from build123d import *

# Parameters (mm, degrees)
SKETCH8_W                       = 35
SKETCH8_H                       = 30
BOSS_EXTRUDE7_DEPTH             = 80
SKETCH10_R                      = 16.5
CUT_EXTRUDE3_DEPTH              = 18.5
CUT_EXTRUDE3_DEPTH_BACK         = 18.5
SKETCH11_W                      = 38.336381606
SKETCH11_H                      = 16.50007926
CUT_EXTRUDE4_DEPTH              = 18.5
CUT_EXTRUDE4_DEPTH_BACK         = 18.5
SKETCH12_W                      = 33.824881692
SKETCH12_H                      = 15
CUT_EXTRUDE5_DEPTH              = 18.5
CUT_EXTRUDE5_DEPTH_BACK         = 18.5
SKETCH13_W                      = 45.541829225
SKETCH13_H                      = 41.48776408
CUT_EXTRUDE6_DEPTH              = 18.5
CUT_EXTRUDE6_DEPTH_BACK         = 18.5
SKETCH15_W                      = 35
SKETCH15_H                      = 7.5
BOSS_EXTRUDE9_DEPTH             = 2
CUT_EXTRUDE7_DEPTH              = 2
SKETCH18_R                      = 3.2
CUT_EXTRUDE10_DEPTH             = 9.24996037
CUT_EXTRUDE10_DEPTH_BACK        = 6.4
CUT_EXTRUDE11_REACH             = 10.25
SKETCH19_R                      = 3.4
CUT_EXTRUDE11_DIRECTION_2_DEPTH = 4.9


with BuildPart() as part:
    # Sketch8 → Boss-Extrude7 (new body)
    with BuildSketch(Plane(origin=(0, 0, 0), x_dir=(1, 0, 0), z_dir=(0, 1, 0))):
        Rectangle(SKETCH8_W, SKETCH8_H)
    extrude(amount=BOSS_EXTRUDE7_DEPTH)

    # Sketch10 → Cut-Extrude3 (cut, two sides)
    with BuildSketch(Plane(origin=(0, 0, 0), x_dir=(0, 0, -1), z_dir=(1, 0, 0))) as cut_extrude3_sk:
        with Locations((0, 40)):
            Circle(SKETCH10_R)
    extrude(amount=CUT_EXTRUDE3_DEPTH, mode=Mode.SUBTRACT)
    extrude(cut_extrude3_sk.sketch, amount=-CUT_EXTRUDE3_DEPTH_BACK, mode=Mode.SUBTRACT)

    # Sketch11 → Cut-Extrude4 (cut, two sides)
    with BuildSketch(Plane(origin=(0, 0, 0), x_dir=(0, 0, -1), z_dir=(1, 0, 0))) as cut_extrude4_sk:
        with Locations((0, 40)):
            Rectangle(SKETCH11_W, SKETCH11_H)
    extrude(amount=CUT_EXTRUDE4_DEPTH, mode=Mode.SUBTRACT)
    extrude(cut_extrude4_sk.sketch, amount=-CUT_EXTRUDE4_DEPTH_BACK, mode=Mode.SUBTRACT)

    # Sketch12 → Cut-Extrude5 (cut, two sides)
    with BuildSketch(Plane(origin=(0, 0, 0), x_dir=(0, 0, -1), z_dir=(1, 0, 0))) as cut_extrude5_sk:
        with Locations((0.439040256, 7.5)):
            Rectangle(SKETCH12_W, SKETCH12_H)
    extrude(amount=CUT_EXTRUDE5_DEPTH, mode=Mode.SUBTRACT)
    extrude(cut_extrude5_sk.sketch, amount=-CUT_EXTRUDE5_DEPTH_BACK, mode=Mode.SUBTRACT)

    # Sketch13 → Cut-Extrude6 (cut, two sides)
    with BuildSketch(Plane(origin=(0, 0, 0), x_dir=(0, 0, -1), z_dir=(1, 0, 0))) as cut_extrude6_sk:
        with Locations((-6.569234617, 60.808180877)):
            Rectangle(SKETCH13_W, SKETCH13_H)
    extrude(amount=CUT_EXTRUDE6_DEPTH, mode=Mode.SUBTRACT)
    extrude(cut_extrude6_sk.sketch, amount=-CUT_EXTRUDE6_DEPTH_BACK, mode=Mode.SUBTRACT)

    # Sketch15 → Boss-Extrude9 (add)
    with BuildSketch(Plane(origin=(0, 15, 0), x_dir=(-1, 0, 0), z_dir=(0, -1, 0))):
        with Locations((0, -18.75)):
            Rectangle(SKETCH15_W, SKETCH15_H)
        with Locations((0, 18.75)):
            Rectangle(SKETCH15_W, SKETCH15_H)
    extrude(amount=-BOSS_EXTRUDE9_DEPTH)

    # Sketch16 → Cut-Extrude7 (cut)
    with BuildSketch(Plane(origin=(0, 15, 0), x_dir=(-1, 0, 0), z_dir=(0, -1, 0))):
        with BuildLine():
            Line((10, -20.863517543), (-10, -20.863517543))
            ThreePointArc((-10, -20.863517543), (-12, -18.863517543), (-10, -16.863517543))
            Line((-10, -16.863517543), (10, -16.863517543))
            ThreePointArc((10, -16.863517543), (12, -18.863517543), (10, -20.863517543))
        make_face()
        with BuildLine():
            Line((10, 16.803450623), (-10, 16.803450623))
            ThreePointArc((-10, 16.803450623), (-12, 18.803450623), (-10, 20.803450623))
            Line((-10, 20.803450623), (10, 20.803450623))
            ThreePointArc((10, 20.803450623), (12, 18.803450623), (10, 16.803450623))
        make_face()
    extrude(amount=-CUT_EXTRUDE7_DEPTH, mode=Mode.SUBTRACT)

    # Sketch18 → Cut-Extrude10 (cut, two sides)
    with BuildSketch(Plane(origin=(0, 23.5, 0), x_dir=(1, 0, 0), z_dir=(0, 1, 0))) as cut_extrude10_sk:
        Circle(SKETCH18_R)
        with Locations((10, 0)):
            Circle(SKETCH18_R)
        with Locations((-10, 0)):
            Circle(SKETCH18_R)
    extrude(amount=CUT_EXTRUDE10_DEPTH, mode=Mode.SUBTRACT)
    extrude(cut_extrude10_sk.sketch, amount=-CUT_EXTRUDE10_DEPTH_BACK, mode=Mode.SUBTRACT)

    # Sketch19 → Cut-Extrude11 (cut, up to next)
    with BuildSketch(Plane(origin=(0, 23.5, 0), x_dir=(1, 0, 0), z_dir=(0, 1, 0)), mode=Mode.PRIVATE) as cut_extrude11_sk1:
        with Locations((-10, -10)):
            Circle(SKETCH19_R)
    cut_extrude11_tool1 = extrude(cut_extrude11_sk1.sketch, amount=CUT_EXTRUDE11_REACH, mode=Mode.PRIVATE) & part.part
    add(cut_extrude11_tool1.solids().sort_by_distance((-10, 23.5, 10))[0], mode=Mode.SUBTRACT)
    # Sketch19 → Cut-Extrude11 (cut, up to next)
    with BuildSketch(Plane(origin=(0, 23.5, 0), x_dir=(1, 0, 0), z_dir=(0, 1, 0)), mode=Mode.PRIVATE) as cut_extrude11_sk2:
        with Locations((0, -10)):
            Circle(SKETCH19_R)
    cut_extrude11_tool2 = extrude(cut_extrude11_sk2.sketch, amount=CUT_EXTRUDE11_REACH, mode=Mode.PRIVATE) & part.part
    add(cut_extrude11_tool2.solids().sort_by_distance((0, 23.5, 10))[0], mode=Mode.SUBTRACT)
    # Sketch19 → Cut-Extrude11 (cut, up to next)
    with BuildSketch(Plane(origin=(0, 23.5, 0), x_dir=(1, 0, 0), z_dir=(0, 1, 0)), mode=Mode.PRIVATE) as cut_extrude11_sk3:
        with Locations((10, -10)):
            Circle(SKETCH19_R)
    cut_extrude11_tool3 = extrude(cut_extrude11_sk3.sketch, amount=CUT_EXTRUDE11_REACH, mode=Mode.PRIVATE) & part.part
    add(cut_extrude11_tool3.solids().sort_by_distance((10, 23.5, 10))[0], mode=Mode.SUBTRACT)
    # Sketch19 → Cut-Extrude11 (cut, up to next)
    with BuildSketch(Plane(origin=(0, 23.5, 0), x_dir=(1, 0, 0), z_dir=(0, 1, 0)), mode=Mode.PRIVATE) as cut_extrude11_sk4:
        with Locations((-10, 10)):
            Circle(SKETCH19_R)
    cut_extrude11_tool4 = extrude(cut_extrude11_sk4.sketch, amount=CUT_EXTRUDE11_REACH, mode=Mode.PRIVATE) & part.part
    add(cut_extrude11_tool4.solids().sort_by_distance((-10, 23.5, -10))[0], mode=Mode.SUBTRACT)
    # Sketch19 → Cut-Extrude11 (cut, up to next)
    with BuildSketch(Plane(origin=(0, 23.5, 0), x_dir=(1, 0, 0), z_dir=(0, 1, 0)), mode=Mode.PRIVATE) as cut_extrude11_sk5:
        with Locations((0, 10)):
            Circle(SKETCH19_R)
    cut_extrude11_tool5 = extrude(cut_extrude11_sk5.sketch, amount=CUT_EXTRUDE11_REACH, mode=Mode.PRIVATE) & part.part
    add(cut_extrude11_tool5.solids().sort_by_distance((0, 23.5, -10))[0], mode=Mode.SUBTRACT)
    # Sketch19 → Cut-Extrude11 (cut, up to next)
    with BuildSketch(Plane(origin=(0, 23.5, 0), x_dir=(1, 0, 0), z_dir=(0, 1, 0)), mode=Mode.PRIVATE) as cut_extrude11_sk6:
        with Locations((10, 10)):
            Circle(SKETCH19_R)
    cut_extrude11_tool6 = extrude(cut_extrude11_sk6.sketch, amount=CUT_EXTRUDE11_REACH, mode=Mode.PRIVATE) & part.part
    add(cut_extrude11_tool6.solids().sort_by_distance((10, 23.5, -10))[0], mode=Mode.SUBTRACT)

    # Sketch19 → Cut-Extrude11 direction 2 (cut)
    with BuildSketch(Plane(origin=(0, 23.5, 0), x_dir=(1, 0, 0), z_dir=(0, 1, 0))):
        with Locations((-10, -10)):
            Circle(SKETCH19_R)
        with Locations((0, -10)):
            Circle(SKETCH19_R)
        with Locations((10, -10)):
            Circle(SKETCH19_R)
        with Locations((-10, 10)):
            Circle(SKETCH19_R)
        with Locations((0, 10)):
            Circle(SKETCH19_R)
        with Locations((10, 10)):
            Circle(SKETCH19_R)
    extrude(amount=-CUT_EXTRUDE11_DIRECTION_2_DEPTH, mode=Mode.SUBTRACT)


solid = part.part
The listing builds one solid part. Answer for the finished solid, in the listing's coordinates (mm). A direction names the side the tool comes from. Give positions to 0.01 mm unless a question says otherwise; leave off trailing zeros. Loops run counter-clockwise (first coordinate to the right, second up) from the corner with the lowest first, then second, coordinate; pieces in that order, holes last.
Item 1: Each of these flat-tipped pins is pushed along its axis until it touches: pin 1 Ø1.9 at (x, z) = (-11, -1.5) entering from +Y; pin 2 Ø1 at (x, z) = (6, 1) entering from +Y; pin 3 Ø6 at (x, z) = (-6.5, 20) entering from +Y. Where does it stop, or does it pass through?
Derived:
pin 1: stops at y = 17.1
pin 2: stops at y = 23.57
pin 3: stops at y = 17
Item 2: A cutting plane is placed at A-A (x = -5.5). Give the vertices of the cut face in (y, z).
Derived:
outline: (15, -22.5) - (17, -22.5) - (17, -20.8) - (15, -20.8) - close; (15, -16.8) - (17, -16.8) - (17, -15) - (31.75, -15) - (31.75, -14.29) arc R16.5 cw to (31.75, 14.29) - (31.75, 15) - (17, 15) - (17, 16.86) - (15, 16.86) - close; (15, 20.86) - (17, 20.86) - (17, 22.5) - (15, 22.5) - close
Item 3: Determine the mould class of faces 1 (the flat face through (-17.5, 21, -5)), 2 (the flat face through (0, 16, 20.864)), 3 (the flat face through (0, 16, 22.5)) for opening direction X: +X half, -X half, draft (parallel to the pull), parting line (faces both ways), or undercut.
Derived:
face 1: -X half
face 2: undercut
face 3: draft
Item 4: A tool of negligible diameter and unlimited length cuts with its end or side. For faces 4 (the cylindrical face through (-12, 16, 18.8)), 5 (the flat face through (0, 17, 16)), 6 (the flat face through (-10, 18.6, 10)), from which of +Z, -Z, +X, -X, +Y, -Y can it reach the whole face along a straight path? Write none if from no direction.
Derived:
face 4: +Y, -Y
face 5: +Z, +X, -X, +Y
face 6: +Y
Item 5: A cutting plane is placed at D-D (z = -1.5). Give the vertices of the cut face in (x, y).
Derived:
outline: (-17.5, 15) - (17.5, 15) - (17.5, 23.57) - (12.83, 23.57) - (12.83, 17.1) - (7.17, 17.1) - (7.17, 23.57) - (2.83, 23.57) - (2.83, 17.1) - (-2.83, 17.1) - (-2.83, 23.57) - (-7.17, 23.57) - (-7.17, 17.1) - (-12.83, 17.1) - (-12.83, 23.57) - (-17.5, 23.57) - close
Item 6: A cutting plane is placed at B-B (y = 24.75). Give the vertices of the cut face in (x, z).
Derived:
outline: (-17.5, -15) - (17.5, -15) - (17.5, -6.3) - (-17.5, -6.3) - close; (-17.5, 6.3) - (17.5, 6.3) - (17.5, 15) - (-17.5, 15) - close; hole circle Ø6.8 at (-10, -10); hole circle Ø6.8 at (-10, 10); hole circle Ø6.8 at (0, -10); hole circle Ø6.8 at (0, 10); hole circle Ø6.8 at (10, -10); hole circle Ø6.8 at (10, 10)
Item 7: Find the intervals of material crossed by line 1 along Z through (x, y) = (0, 22.3); line 2 along X through (y, z) = (25, -10); line 3 along X through (y, z) = (19.75, 0), in increasing order.
Derived:
line 1: z = -15 to -13.4, -6.6 to -3.2, 3.2 to 6.6, 13.4 to 15
line 2: x = -17.5 to -13.4, -6.6 to -3.4, 3.4 to 6.6, 13.4 to 17.5
line 3: x = -17.5 to -13.2, -6.8 to -3.2, 3.2 to 6.8, 13.2 to 17.5
Item 8: A cutting plane is placed at C-C (y = 29.25). Give the vertices of the cut face in (x, z), then the cut area to 3 significant figures.
Derived:
outline: (-17.5, -15) - (17.5, -15) - (17.5, -12.52) - (12.29, -12.52) arc R3.4 cw to (7.71, -12.52) - (2.29, -12.52) arc R3.4 cw to (-2.29, -12.52) - (-7.71, -12.52) arc R3.4 cw to (-12.29, -12.52) - (-17.5, -12.52) - close; (-17.5, 12.52) - (-12.29, 12.52) arc R3.4 cw to (-7.71, 12.52) - (-2.29, 12.52) arc R3.4 cw to (2.29, 12.52) - (7.71, 12.52) arc R3.4 cw to (12.29, 12.52) - (17.5, 12.52) - (17.5, 15) - (-17.5, 15) - close
area: 157 mm2
